```python
from build123d import *

# Parameters (mm, degrees)
SKETCH1_R               = 3.4925
BOSS_EXTRUDE1_DEPTH     = 23.8125
SKETCH2_R               = 4.7625
BOSS_EXTRUDE2_DEPTH     = 1.5875
CUT_EXTRUDE1_DEPTH      = 27.277800755
CUT_EXTRUDE1_DEPTH_BACK = 27.277800755
SKETCH3_R               = 1.058333333
FILLET1_R               = 0.1984375
FILLET3_R               = 0.79375
CHAMFER1_SIZE           = 0.79375
FILLET4_R               = 0.396875


with BuildPart() as part:
    # Sketch1 → Boss-Extrude1 (new body)
    with BuildSketch(Plane.XY):
        Circle(SKETCH1_R)
    extrude(amount=BOSS_EXTRUDE1_DEPTH)

    # Sketch2 → Boss-Extrude2 (add)
    with BuildSketch(Plane.XY.offset(23.8125)):
        Circle(SKETCH2_R)
    extrude(amount=BOSS_EXTRUDE2_DEPTH)

    # Sketch3 → Cut-Extrude1 (cut, two sides: drawn at the far end of the back side and taken through both)
    with BuildSketch(Plane(origin=(0, 0, 0), x_dir=(1, 0, 0), z_dir=(0, 1, 0)).offset(-CUT_EXTRUDE1_DEPTH_BACK)):
        with Locations(Location((0, -3.429, 0), (0, 0, 270))):
            Circle(SKETCH3_R)
    extrude(amount=CUT_EXTRUDE1_DEPTH + CUT_EXTRUDE1_DEPTH_BACK, mode=Mode.SUBTRACT)

    # Fillet1
    fillet1_edges = [part.edges().sort_by_distance(p)[0] for p in [
        (0, 3.492500015, 2.370666678),
        (0, -3.492500015, 2.370666678),
    ]]
    fillet(fillet1_edges, radius=FILLET1_R)

    # Fillet3
    fillet3_edges = [part.edges().sort_by_distance(p)[0] for p in [
        (-4.7625, 0, 23.8125),
    ]]
    fillet(fillet3_edges, radius=FILLET3_R)

    # Chamfer1
    chamfer1_edges = [part.edges().sort_by_distance(p)[0] for p in [
        (-3.4925, 0, 0),
    ]]
    chamfer(chamfer1_edges, length=CHAMFER1_SIZE)

    # Fillet4
    fillet4_edges = [part.edges().sort_by_distance(p)[0] for p in [
        (-3.4925, 0, 0.79375),
        (-2.69875, 0, 0),
    ]]
    fillet(fillet4_edges, radius=FILLET4_R)


solid = part.part
```
Here's how the part is built. I have some questions about the finished solid (model axes, mm). Coordinates: 2 decimals unless noted, no trailing zeros. Write each loop counter-clockwise with the first axis right and the second up, starting at its lowest first coordinate (ties: lowest second). Pieces come first, ordered by that corner, then holes. Notation, with made-up numbers: (41, 62) -> (59, 62) arc R25 cw to (59, 101) -> close; hole circle Ø3 at (-13.5, -21). An arc over 180 degrees is marked (long way). Use a Markdown table: item, result. Add a question column.
(1) I'm going to push flat-ended pins straight in: P1, Ø1, axis at y = -0.5, z = 6.5, coming from the -X side; P2, Ø1.3, axis at x = 0, z = 3.429, coming from the -Y side; P3, Ø2, axis at x = 1, z = 21.5, coming from the -Y side; P4, Ø3, axis at x = -3.5, z = 6.5, coming from the -Y side. Where does each tip first touch, or does it pass through?
(2) If we section it at A-A, the plane z = 10: Write out the boundary of the cut face in (x, y) (1 decimal).
(3) Please list where these lines run through material, in increasing order: line 1 (Z direction, x = 0, y = 1.25); line 2 (X direction, y = 1.5, z = 3.25); line 3 (Y direction, x = 0, z = 15.5).
(4) We'd pull the mould along X, two halves only. Please class faces 1 (the flat face through (0, 0, 25.4)), 2 (the cylindrical face through (-0.8, -3.4, 12.2)), 3 (the cylindrical face through (0.318, -0.046, 4.438)): +X half, -X half, draft (parallel to the pull), parting line (faces both ways), or undercut.
Outcome:
| question | item | result |
|---|---|---|
| 1 | P1 | stops at x = -3.49 |
| 1 | P2 | passes through |
| 1 | P3 | stops at y = -3.49 |
| 1 | P4 | stops at y = -2.86 |
| 2 | outline | circle Ø7 at (0, 0) |
| 3 | line 1 | z = 0 to 2.37, 4.49 to 25.4 |
| 3 | line 2 | x = -3.15 to -1.04, 1.04 to 3.15 |
| 3 | line 3 | y = -3.49 to 3.49 |
| 4 | face 1 | draft |
| 4 | face 2 | parting line |
| 4 | face 3 | undercut |
